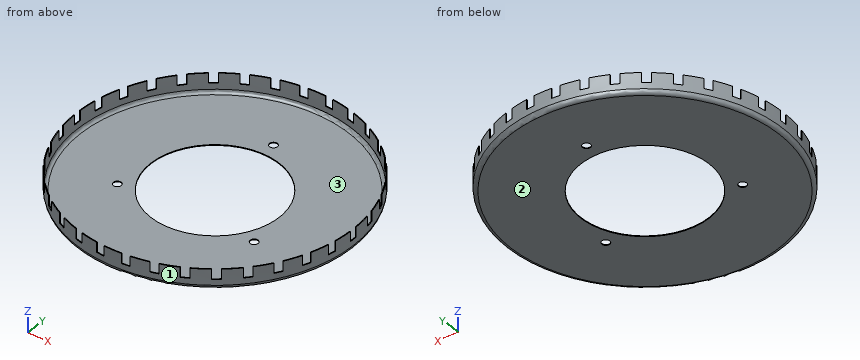
```python
from build123d import *

# Parameters (mm, degrees)
SKETCH1_R                  = 88.9
EXTRUDE1_DEPTH             = 12.7
FILLET1_R                  = 2.54
SHELL1_T                   = -0.508
F_1_1_DIAMETER_HOLE1_D     = 82.55
F_1_1_DIAMETER_HOLE1_DEPTH = 17.78
F_1_1_DIAMETER_HOLE1_TIP   = 24.80052205
SKETCH3_W                  = 6.35
SKETCH3_H                  = 5.08
EXTRUDE2_DEPTH             = 127.363404513
CIRPATTERN1_COUNT          = 17
F_10_CLEARANCE_HOLE1_D     = 5.1054
CIRPATTERN2_COUNT          = 3


with BuildPart() as part:
    # Sketch1 → Extrude1 (new body)
    with BuildSketch(Plane.XY):
        Circle(SKETCH1_R)
    extrude(amount=EXTRUDE1_DEPTH)

    # Fillet1
    fillet1_edges = [part.edges().sort_by_distance(p)[0] for p in [
        (-88.9, 0, 0),
    ]]
    fillet(fillet1_edges, radius=FILLET1_R)

    # Shell1
    shell1_openings = [part.faces().sort_by_distance(p)[0] for p in [
        (0, 0, 12.7),
    ]]
    offset(amount=SHELL1_T, openings=shell1_openings, kind=Kind.INTERSECTION)

    # 1 (1) Diameter Hole1
    with Locations(Plane.XY.offset(0.508)):
        with Locations((0, 0)):
            Hole(F_1_1_DIAMETER_HOLE1_D / 2, depth=F_1_1_DIAMETER_HOLE1_DEPTH)
            with Locations((0, 0, -(F_1_1_DIAMETER_HOLE1_DEPTH + F_1_1_DIAMETER_HOLE1_TIP / 2))):  # 118° drill point
                Cone(0, F_1_1_DIAMETER_HOLE1_D / 2, F_1_1_DIAMETER_HOLE1_TIP, mode=Mode.SUBTRACT)

    # Sketch3 → Extrude2 (cut, symmetric)
    with BuildSketch(Plane(origin=(0, 0, 0), x_dir=(0, 0, -1), z_dir=(1, 0, 0))):
        with Locations((-9.525, 0)):
            Rectangle(SKETCH3_W, SKETCH3_H)
    extrude2 = extrude(amount=EXTRUDE2_DEPTH, both=True, mode=Mode.SUBTRACT)

    # CirPattern1: Extrude2 ×17 about axis
    cirpattern1_axis = Axis((0, 0, 0), (0, 0, 1))
    for i in range(1, CIRPATTERN1_COUNT):
        add(extrude2.rotate(cirpattern1_axis, i * 360 / CIRPATTERN1_COUNT), mode=Mode.SUBTRACT)

    # #10 Clearance Hole1 (through all)
    with Locations(Plane(origin=(0, 50.8, 0.508), x_dir=(1, 0, 0), z_dir=(0, 0, 1))):
        with Locations((0, 0)):
            f_10_clearance_hole1 = Hole(F_10_CLEARANCE_HOLE1_D / 2)

    # CirPattern2: #10 Clearance Hole1 ×3 about axis
    cirpattern2_axis = Axis((0, 0, 0), (0, 0, 1))
    for i in range(1, CIRPATTERN2_COUNT):
        add(f_10_clearance_hole1.rotate(cirpattern2_axis, i * 360 / CIRPATTERN2_COUNT), mode=Mode.SUBTRACT)


solid = part.part
```
Could you check a few things on this model? Use its own coordinates, in mm. Face numbers are marked on the shaded views. Give positions to 0.01 mm unless a question says otherwise; leave off trailing zeros. Loops run counter-clockwise (first coordinate to the right, second up) from the corner with the lowest first, then second, coordinate; pieces in that order, holes last. Notation, with made-up numbers: (47, 77.5) -> (61, 77.5) arc R13 cw to (61, 82.5) -> close; hole circle Ø10 at (22.25, -30). An arc over 180 degrees is marked (long way). Put each result on its own line as item: value.
(1) Imagine slicing it at B-B on z = 9.5. State how many separate pieces and enclosed holes the cut face has, plus the area to 3 significant figures.
Computed:
separate pieces: 34
enclosed holes: 0
area: 195 mm^2
(2) I'm going to push flat-ended pins straight in: pin 1 Ø6 at (y, z) = (-52.5, 9.5) entering from +X; pin 2 Ø0.9 at (x, y) = (74.5, -47) entering from +Z; pin 3 Ø1.5 at (x, z) = (-64, 9.5) entering from -Y. Where does each tip first touch, or does it pass through?
Computed:
pin 1: x = 73.84
pin 2: z = 6.35
pin 3: y = -62.47
(3) Thinking about a two-plate mould opening in X: for the marked faces 1, 2 and 3, which applies, pulls with the +X half, pulls with the -X half, needs draft (parallel to the pull), parting line crosses it, or undercut?
Computed:
face 1: parting line crosses it
face 2: needs draft
face 3: undercut
(4) Please list where these lines run through material, in increasing order: probe 1 along Y at (x, z) = (0, 0.4) (3 decimals); probe 2 along Y at (x, z) = (0, 0.45) (3 decimals); probe 3 along Y at (x, z) = (-19, 4). Write a range as [from, to].
Computed:
probe 1: [-87.728, -41.275], [41.275, 48.247], [53.353, 87.728]
probe 2: [-87.803, -41.275], [41.275, 48.247], [53.353, 87.803]
probe 3: [-86.85, -86.33], [86.33, 86.85]
(5) Imagine slicing it at A-A on y = 0. Write out the boundary of the cut face in (x, z) (3 decimals), plus the area to 3 significant figures.
Computed:
outline: (-88.9, 2.54) arc R2.54 ccw to (-86.36, 0) -> (-41.275, 0) -> (-41.275, 0.508) -> (-86.36, 0.508) arc R2.032 cw to (-88.392, 2.54) -> (-88.392, 6.35) -> (-88.9, 6.35) -> close; (41.275, 0) -> (86.36, 0) arc R2.54 ccw to (88.9, 2.54) -> (88.9, 6.35) -> (88.392, 6.35) -> (88.392, 2.54) arc R2.032 cw to (86.36, 0.508) -> (41.275, 0.508) -> close
area: 53.3 mm^2
